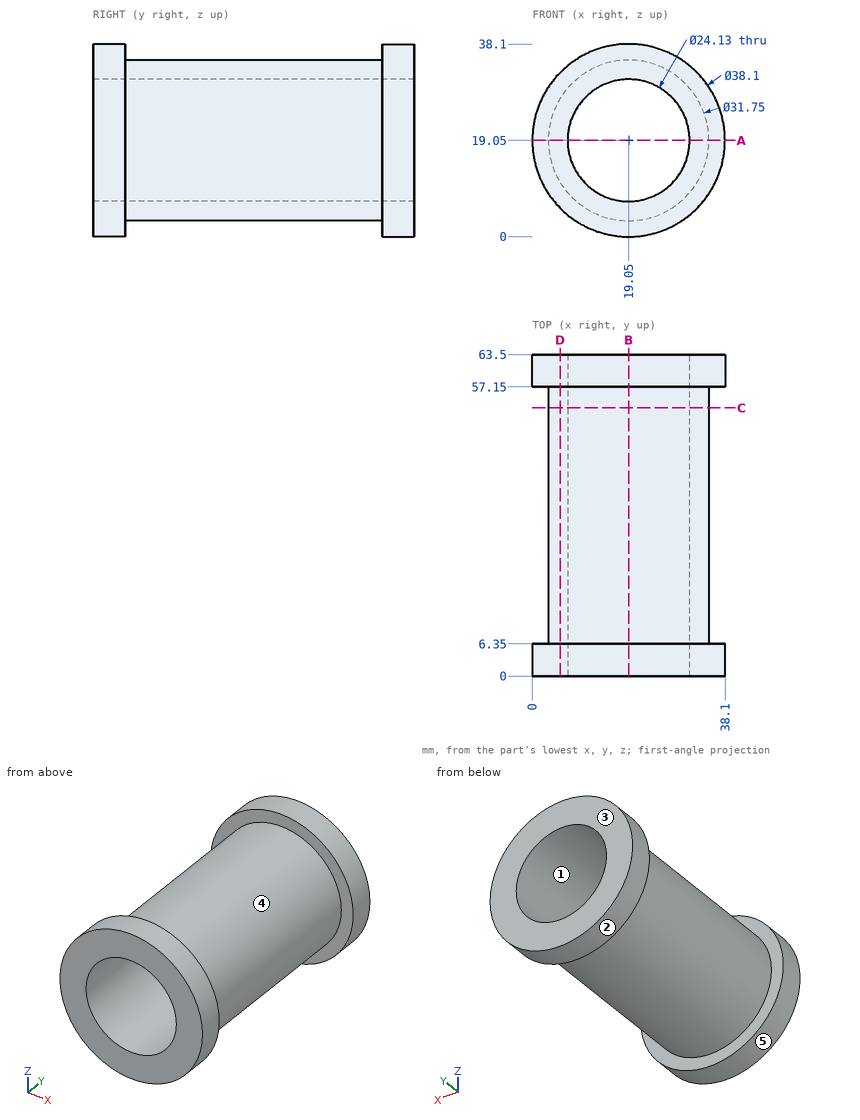
Verification items for this drawing (mm, ordinates from the low corner). A direction names the side the tool comes from. Round coordinates to 2 decimals unless told otherwise and drop trailing zeros. Loops run counter-clockwise (first coordinate to the right, second up) from the corner with the lowest first, then second, coordinate; pieces in that order, holes last. Notation, with made-up numbers: (54.5, -13) -> (113.5, -13) arc R28 ccw to (113.5, 25) -> close; hole circle Ø6 at (-22, -33.5). An arc over 180 degrees is marked (long way). Write item = value, one per line. Start each with the question number.
1) Release check for a two-part mould opening along Z. For the marked faces 1, 2 and 3 record: released by +Z, released by -Z, zero draft, split by the parting line, or undercut.
2) Sectioned sample at A-A, the plane z = 19.05. Record the cut outline in (x, y) (3 decimals).
3) Set-up check for the marked faces 4 and 5: record each of +Z, -Z, +X, -X, +Y, -Y from which the full face is reachable in a straight line by a thin tool's end or side.
4) Sectioned sample at B-B, the plane x = 19.05. Record the cut outline in (y, z) (3 decimals).
5) Sectioned sample at C-C, the plane y = 53. Record the cut outline in (x, z) (3 decimals).
6) Sectioned sample at D-D, the plane x = 5.5. Record the cut outline in (y, z).
7) Thickness scan on probe 1 along Z at (x, y) = (19.05, 26.5) (3 decimals); probe 2 along X at (y, z) = (50, 19); probe 3 along Y at (x, z) = (16, 2.5). Record the ranges inside material, lowest first.
8) Gauge pin test, flat ends, axial feed: pin 1 Ø11.5 at (x, z) = (26, 19.5) entering from -Y; pin 2 Ø4 at (y, z) = (36, 34) entering from +X; pin 3 Ø2 at (y, z) = (39, 5.5) entering from -X; pin 4 Ø2 at (y, z) = (33, 6) entering from -X. Record the tip position at first contact, or that the pin passes through.
Results are:
q1.face_1 = undercut
q1.face_2 = split by the parting line
q1.face_3 = zero draft
q2.outline = (0, 0) -> (6.985, 0) -> (6.985, 63.5) -> (0, 63.5) -> (0, 57.15) -> (3.175, 57.15) -> (3.175, 6.35) -> (0, 6.35) -> close; (31.115, 0) -> (38.1, 0) -> (38.1, 6.35) -> (34.925, 6.35) -> (34.925, 57.15) -> (38.1, 57.15) -> (38.1, 63.5) -> (31.115, 63.5) -> close
q3.face_4 = none
q3.face_5 = +Y, -Y
q4.outline = (0, 0) -> (6.35, 0) -> (6.35, 3.175) -> (57.15, 3.175) -> (57.15, 0) -> (63.5, 0) -> (63.5, 6.985) -> (0, 6.985) -> close; (0, 31.115) -> (63.5, 31.115) -> (63.5, 38.1) -> (57.15, 38.1) -> (57.15, 34.925) -> (6.35, 34.925) -> (6.35, 38.1) -> (0, 38.1) -> close
q5.outline = circle Ø31.75 at (19.05, 19.05); hole circle Ø24.13 at (19.05, 19.05)
q6.outline = (0, 5.66) -> (6.35, 5.66) -> (6.35, 10.78) -> (57.15, 10.78) -> (57.15, 5.66) -> (63.5, 5.66) -> (63.5, 32.44) -> (57.15, 32.44) -> (57.15, 27.32) -> (6.35, 27.32) -> (6.35, 32.44) -> (0, 32.44) -> close
q7.probe_1 = 3.175 to 6.985, 31.115 to 34.925
q7.probe_2 = 3.18 to 6.99, 31.11 to 34.92
q7.probe_3 = 0 to 6.35, 57.15 to 63.5
q8.pin_1 = 0
q8.pin_2 = 28.23
q8.pin_3 = 9.33
q8.pin_4 = 8.71
